from build123d import *

# Parameters (mm, degrees)
SALIENTE_EXTRUIR1_DEPTH = 100
CROQUIS2_W              = 13
CROQUIS2_H              = 28.5
CORTAR_EXTRUIR2_DEPTH   = 10
CROQUIS3_R              = 1.5
CORTAR_EXTRUIR3_DEPTH   = 5
CROQUIS4_R              = 1.5
CORTAR_EXTRUIR4_DEPTH   = 10
CROQUIS5_R              = 1.5
CORTAR_EXTRUIR6_DEPTH   = 10


with BuildPart() as part:
    # Croquis1 → Saliente-Extruir1 (new body)
    with BuildSketch(Plane.XY):
        Polygon((50, 0), (-50, 0), (-50, 50), (-47, 50), (-47, 2.5), (47, 2.5), (47, 50), (50, 50), align=None)
    extrude(amount=-SALIENTE_EXTRUIR1_DEPTH)

    # Croquis2 → Cortar-Extruir2 (cut)
    with BuildSketch(Plane(origin=(0, 2.5, 0), x_dir=(1, 0, 0), z_dir=(0, 1, 0))):
        with Locations((-40.5, 14.25)):
            Rectangle(CROQUIS2_W, CROQUIS2_H)
        with Locations((40.5, 14.25)):
            Rectangle(CROQUIS2_W, CROQUIS2_H)
    extrude(amount=-CORTAR_EXTRUIR2_DEPTH, mode=Mode.SUBTRACT)

    # Croquis3 → Cortar-Extruir3 (cut)
    with BuildSketch(Plane(origin=(0, 2.5, 0), x_dir=(1, 0, 0), z_dir=(0, 1, 0))):
        with Locations(Location((0, 5, 0), (0, 0, 270))):
            Circle(CROQUIS3_R)
    extrude(amount=-CORTAR_EXTRUIR3_DEPTH, mode=Mode.SUBTRACT)

    # Croquis4 → Cortar-Extruir4 (cut)
    with BuildSketch(Plane(origin=(0, 2.5, 0), x_dir=(1, 0, 0), z_dir=(0, 1, 0))):
        with Locations(Location((-8.5, 17.75, 0), (0, 0, 270))):
            Circle(CROQUIS4_R)
        with Locations(Location((-8.5, 10.75, 0), (0, 0, 270))):
            Circle(CROQUIS4_R)
        with Locations(Location((8.5, 10.75, 0), (0, 0, 180))):
            Circle(CROQUIS4_R)
        with Locations(Location((8.5, 17.75, 0), (0, 0, 180))):
            Circle(CROQUIS4_R)
    extrude(amount=-CORTAR_EXTRUIR4_DEPTH, mode=Mode.SUBTRACT)

    # Croquis5 → Cortar-Extruir6 (cut)
    with BuildSketch(Plane(origin=(0, 2.5, 0), x_dir=(1, 0, 0), z_dir=(0, 1, 0))):
        with Locations(Location((-24, 89.05, 0), (0, 0, 270))):
            Circle(CROQUIS5_R)
        with Locations(Location((-24, 33.05, 0), (0, 0, 270))):
            Circle(CROQUIS5_R)
        with Locations(Location((24, 33.05, 0), (0, 0, 180))):
            Circle(CROQUIS5_R)
        with Locations(Location((24, 89.05, 0), (0, 0, 180))):
            Circle(CROQUIS5_R)
    extrude(amount=-CORTAR_EXTRUIR6_DEPTH, mode=Mode.SUBTRACT)


solid = part.part
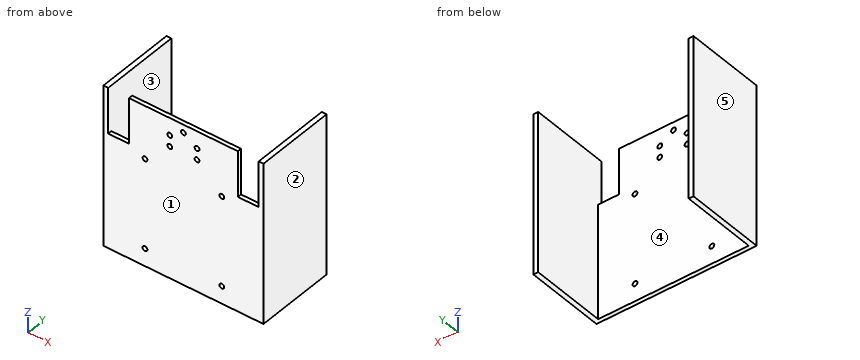
The listing builds one solid part. Answer for the finished solid, in the listing's coordinates (mm). Face numbers are marked on the shaded views. A direction names the side the tool comes from. Round coordinates to 2 decimals unless told otherwise and drop trailing zeros. Order: outer loops, then holes, each group sorted by start corner. A loop starts at its lowest first (then second) coordinate and runs counter-clockwise, first axis right, second up. Notation, with made-up numbers: (41.25, 69) -> (60.25, 69) arc R20 cw to (60.25, 88) -> close; hole circle Ø8 at (-11, 58.25). An arc over 180 degrees is marked (long way). Write each question's results on one line, items separated by ' | '. Start each with the question number.
Q1. Each of these flat-tipped pins is pushed along its axis until it touches: pin 1 (6 mm diameter, centred on x = -38.5, z = -81.5, fed in from +Y); pin 2 (0.8 mm diameter, centred on x = -38, y = 2, fed in from +Z). Where does it stop, or does it pass through?
Q2. Find section D-D (y = 36). Determine the outline of the cut face in (x, z).
Q3. Find section A-A (z = -10.75). Determine the outline of the cut face in (x, y), then the cut area to 3 significant figures.
Q4. Find section B-B (x = 24). Determine the outline of the cut face in (y, z), then the cut area to 3 significant figures.
Q5. Which of the six approach directions +Z, -Z, +X, -X, +Y, -Y give full straight-line access (tool end or side, diameter ignored) to the marked faces 4 and 5?
Q6. The mould has two halves that part along X. Classify the marked faces 1, 2 and 3: pulls with the +X half, pulls with the -X half, needs draft (parallel to the pull), parting line crosses it, or undercut.
Q7. Straight lines are drawn through the part: probe 1 along X at (y, z) = (1.8, -89.05); probe 2 along X at (y, z) = (46, -9); probe 3 along Z at (x, y) = (8, 1). For each, find the intervals that lie inside material, in ascending order. Write a range as from..to.
Q8. Find section C-C (z = -33.05). Determine the outline of the cut face in (x, y), then the cut area to 3 significant figures.
Worked answers:
1) pin 1: stops at y = 2.5 | pin 2: stops at z = -28.5
2) outline: (-50, -100) -> (-47, -100) -> (-47, 0) -> (-50, 0) -> close; (47, -100) -> (50, -100) -> (50, 0) -> (47, 0) -> close
3) outline: (-50, 0) -> (-47, 0) -> (-47, 50) -> (-50, 50) -> close; (-34, 0) -> (-10, 0) -> (-10, 2.5) -> (-34, 2.5) -> close; (-7, 0) -> (7, 0) -> (7, 2.5) -> (-7, 2.5) -> close; (10, 0) -> (34, 0) -> (34, 2.5) -> (10, 2.5) -> close; (47, 0) -> (50, 0) -> (50, 50) -> (47, 50) -> close | area: 455 mm2
4) outline: (0, -100) -> (2.5, -100) -> (2.5, -90.55) -> (0, -90.55) -> close; (0, -87.55) -> (2.5, -87.55) -> (2.5, -34.55) -> (0, -34.55) -> close; (0, -31.55) -> (2.5, -31.55) -> (2.5, 0) -> (0, 0) -> close | area: 235 mm2
5) face 4: +Z, -Z, +Y | face 5: +Z, -Z, -X, +Y, -Y
6) face 1: needs draft | face 2: pulls with the +X half | face 3: undercut
7) probe 1: x = -50..-25.5, -22.5..22.5, 25.5..50 | probe 2: x = -50..-47, 47..50 | probe 3: z = -100..-19.16, -16.34..-12.16, -9.34..0
8) outline: (-50, 0) -> (-25.5, 0) -> (-25.5, 2.5) -> (-47, 2.5) -> (-47, 50) -> (-50, 50) -> close; (-22.5, 0) -> (22.5, 0) -> (22.5, 2.5) -> (-22.5, 2.5) -> close; (25.5, 0) -> (50, 0) -> (50, 50) -> (47, 50) -> (47, 2.5) -> (25.5, 2.5) -> close | area: 520 mm2
